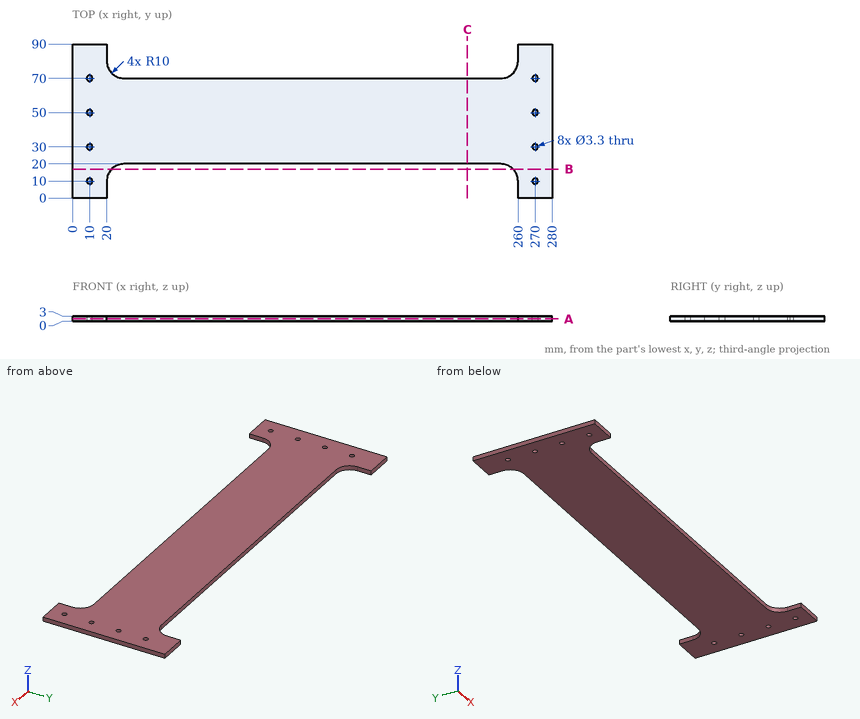
Input: dimensioned drawing with shaded views. Units: mm. Origin: part minimum x, y, z. Coordinates: 2 decimals unless noted, no trailing zeros. Order: outer loops, then holes, each group sorted by start corner. A loop starts at its lowest first (then second) coordinate and runs counter-clockwise, first axis right, second up. Notation, with made-up numbers: (7, 55.5) - (14, 55.5) arc R7 cw to (14, 59.5) - close; hole circle Ø6 at (87, 42). An arc over 180 degrees is marked (long way). Return JSON: item names as keys, results as strings. Group by question number.
1. Material intervals for line 1 along Y through (x, z) = (270, 0.95); line 2 along X through (y, z) = (8, 1.55); line 3 along X through (y, z) = (49.5, 0.45), sorted ascending. Write a range as [from, to].
2. Pin query (flat end, axial travel): pin 1 (2 mm diameter, centred on x = 226.5, y = 36.5, fed in from -Z); pin 2 (3 mm diameter, centred on x = 10, y = 50, fed in from +Z). Return the tip coordinate at first contact, or that it passes through.
3. Cut plane A-A (z = 1.5). Count the separate pieces of the cut face and the enclosed holes in it, plus the area to 3 significant figures.
4. Cut plane B-B (y = 17). Output: boundary loops of the cut face in (x, z).
5. Cut plane C-C (x = 230.5). Output: boundary loops of the cut face in (y, z), plus the area to 3 significant figures.
Resolved:
{
 "1": {"line 1": "y = [0, 8.35], [11.65, 28.35], [31.65, 48.35], [51.65, 68.35], [71.65, 90]", "line 2": "x = [0, 20], [260, 280]", "line 3": "x = [0, 8.43], [11.57, 268.43], [271.57, 280]"},
 "2": {"pin 1": "stops at z = 0", "pin 2": "passes through"},
 "3": {"separate pieces": "1", "enclosed holes": "8", "area": "15,600 mm²"},
 "4": {"outline": "(0, 0) - (22.86, 0) - (22.86, 3) - (0, 3) - close; (257.14, 0) - (280, 0) - (280, 3) - (257.14, 3) - close"},
 "5": {"outline": "(20, 0) - (70, 0) - (70, 3) - (20, 3) - close", "area": "150 mm²"}
}
